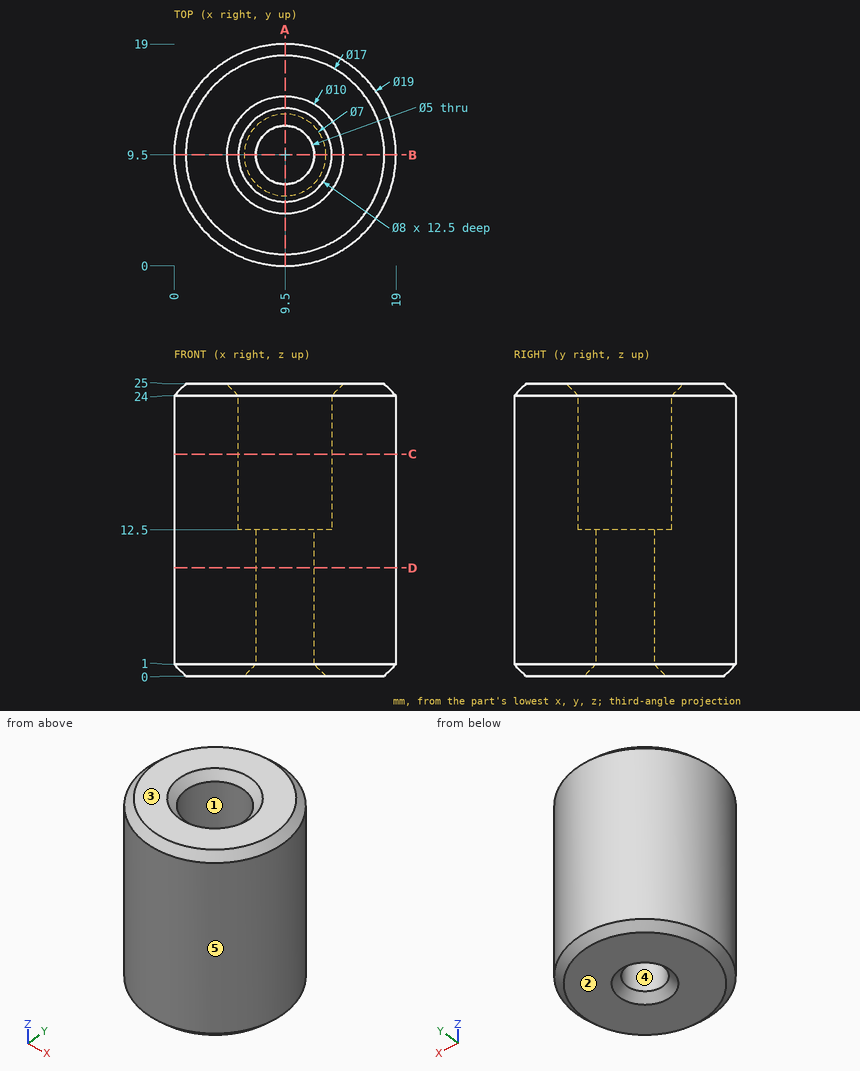
Can you work these out from the drawing? Everything is in mm from the part's minimum corner. A direction names the side the tool comes from. Give positions to 0.01 mm unless a question says otherwise; leave off trailing zeros. Loops run counter-clockwise (first coordinate to the right, second up) from the corner with the lowest first, then second, coordinate; pieces in that order, holes last. Notation, with made-up numbers: M 55,-39 L 73,-39 A22 cw 73,-1 Z; hole C 80,-2.75 d6. An arc over 180 degrees is marked long. Put each result on its own line as item: value. Start each with the question number.
(1) I want a section at D-D on z = 9.25. Please give me the cut outline in (x, y).
(2) I need wall thicknesses on line 1 along Y through (x, z) = (9.5, 20.25); line 2 along X through (y, z) = (9.25, 15.5); line 3 along Y through (x, z) = (9.5, 4.25). Which ranges of each line are inside material? Lowest first, please. Write a range as [from, to].
(3) I want a section at C-C on z = 19. Please give me the cut outline in (x, y), then the cut area to 3 significant figures.
(4) If we mould it in two halves opening along Y, with no side actions, what happens to the marked faces 3, 4 and 5? For each: +Y half, -Y half, draft (parallel to the pull), parting line (faces both ways), or undercut.
(5) Will these pins go through, and if not, where does the flat tip stop? pin 1 Ø1.5 at (x, z) = (14, 12.5) entering from +Y; pin 2 Ø4 at (x, y) = (9.5, 9.5) entering from +Z; pin 3 Ø6 at (y, z) = (15, 19) entering from +X; pin 4 Ø1.5 at (y, z) = (3.5, 4.5) entering from +X.
(6) For the marked faces 1 and 2, which set-ups out of +Z, -Z, +X, -X, +Y, -Y let a thin tool reach every point of the face, with its end or its side?
(7) I want a section at A-A on x = 9.5. Please give me the cut outline in (y, z), then the cut area to 4 significant figures.
Answer block:
1. outline: C 9.5,9.5 d19; hole C 9.5,9.5 d5
2. line 1: [0, 5.5], [13.5, 19]
2. line 2: [0, 5.51], [13.49, 19]
2. line 3: [0, 7], [12, 19]
3. outline: C 9.5,9.5 d19; hole C 9.5,9.5 d8
3. area: 233 mm^2
4. face 3: draft
4. face 4: undercut
4. face 5: parting line
5. pin 1: y = 18.23
5. pin 2: through
5. pin 3: x = 18.67
5. pin 4: x = 17.42
6. face 1: +Z
6. face 2: -Z, +X, -X, +Y, -Y
7. outline: M 0,1 L 1,0 L 6,0 L 7,1 L 7,12.5 L 5.5,12.5 L 5.5,24 L 4.5,25 L 1,25 L 0,24 Z; M 12,1 L 13,0 L 18,0 L 19,1 L 19,24 L 18,25 L 14.5,25 L 13.5,24 L 13.5,12.5 L 12,12.5 Z
7. area: 308.5 mm^2
